```python
from build123d import *

# Parameters (mm, degrees)
SKETCH_1_W         = 42.3
SKETCH_1_H         = 42.3
EXTRUDE_1_DEPTH    = 60
SKETCH_2_R         = 11
EXTRUDE_2_DEPTH    = 2
SKETCH_3_R         = 4
EXTRUDE_3_DEPTH    = 98
HOLE_WIZARD_M3_1_D = 2.5


with BuildPart() as part:
    # 草图1 → 凸台-拉伸1 (new body)
    with BuildSketch(Plane.XY):
        Rectangle(SKETCH_1_W, SKETCH_1_H)
    extrude(amount=EXTRUDE_1_DEPTH)

    # 草图2 → 凸台-拉伸2 (add)
    with BuildSketch(Plane.XY.offset(60)):
        Circle(SKETCH_2_R)
    extrude(amount=EXTRUDE_2_DEPTH)

    # 草图3 → 凸台-拉伸3 (add)
    with BuildSketch(Plane.XY.offset(62)):
        Circle(SKETCH_3_R)
    extrude(amount=EXTRUDE_3_DEPTH)

    # M3 螺纹孔1 (through all)
    with Locations(Plane.XY.offset(60)):
        with Locations((-15.5, 15.5), (15.5, 15.5), (15.5, -15.5), (-15.5, -15.5)):
            Hole(HOLE_WIZARD_M3_1_D / 2)


solid = part.part
```
Can you work these out from the model? Positions are in its coordinate system, mm. A direction names the side the tool comes from. Coordinates: 2 decimals unless noted, no trailing zeros. Loops run counter-clockwise (first coordinate to the right, second up) from the corner with the lowest first, then second, coordinate; pieces in that order, holes last.
1) For pin 1 (3 mm diameter, centred on x = 15.5, y = -15.5, fed in from +Z); pin 2 (10 mm diameter, centred on x = -2, y = -9, fed in from +Z), each with a flat end and sliding along its axis, tell me the tip position at first contact or that it passes through.
2) Imagine slicing it at B-B on x = 6.5. List the corners of the cut face in (y, z) for me, plus the area to 3 significant figures.
3) Which directions (+Z, -Z, +X, -X, +Y, -Y) give clear straight access to the entire face, cutting with the end or side of a thin tool? Please do faces 1 (the flat face through (21.15, 0, 30)), 2 (the cylindrical face through (-0.867, -3.905, 110.314)).
4) Imagine slicing it at D-D on x = 18.5. List the corners of the cut face in (y, z) for me, plus the area to 3 significant figures.
5) Imagine slicing it at A-A on y = 0. List the corners of the cut face in (x, z) for me, plus the area to 3 significant figures.
6) I need wall thicknesses on probe 1 along Y at (x, z) = (15.5, 30); probe 2 along X at (y, z) = (-15, 37); probe 3 along Z at (x, y) = (-16.5, 4). Which ranges of each line are inside material? Lowest first, please.
7) Imagine slicing it at C-C on z = 69.5. List the corners of the cut face in (x, y) for me.
Completed:
1. pin 1: stops at z = 60
1. pin 2: stops at z = 62
2. outline: (-21.15, 0) - (21.15, 0) - (21.15, 60) - (8.87, 60) - (8.87, 62) - (-8.87, 62) - (-8.87, 60) - (-21.15, 60) - close
2. area: 2,570 mm2
3. face 1: +Z, -Z, +X, +Y, -Y
3. face 2: +Z
4. outline: (-21.15, 0) - (21.15, 0) - (21.15, 60) - (-21.15, 60) - close
4. area: 2,540 mm2
5. outline: (-21.15, 0) - (21.15, 0) - (21.15, 60) - (11, 60) - (11, 62) - (4, 62) - (4, 160) - (-4, 160) - (-4, 62) - (-11, 62) - (-11, 60) - (-21.15, 60) - close
5. area: 3,370 mm2
6. probe 1: y = -21.15 to -16.75, -14.25 to 14.25, 16.75 to 21.15
6. probe 2: x = -21.15 to -16.65, -14.35 to 14.35, 16.65 to 21.15
6. probe 3: z = 0 to 60
7. outline: circle Ø8 at (0, 0)
